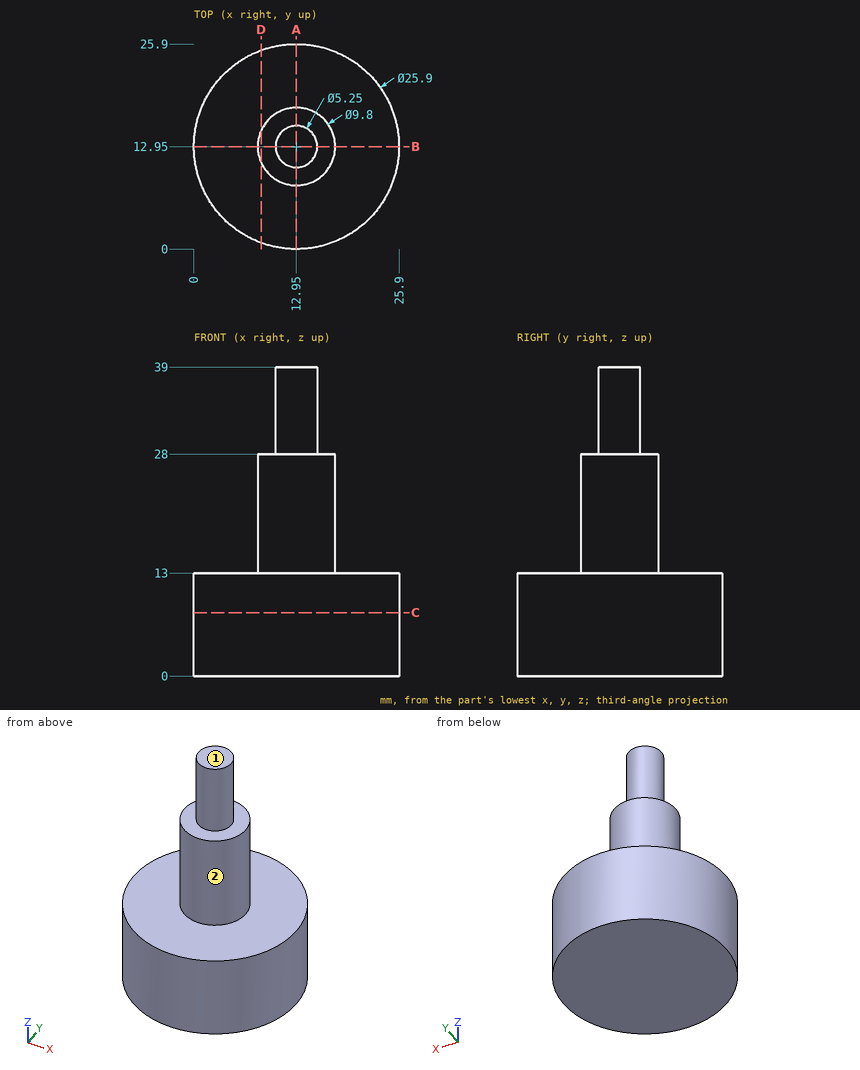
Verification items for this drawing (mm, ordinates from the low corner). A direction names the side the tool comes from. Give positions to 0.01 mm unless a question says otherwise; leave off trailing zeros. Loops run counter-clockwise (first coordinate to the right, second up) from the corner with the lowest first, then second, coordinate; pieces in that order, holes last. Notation, with made-up numbers: M -12,23.5 L 31,23.5 A22 cw 31,47.5 Z; hole C -39,-18.75 d6. An arc over 180 degrees is marked long. Return JSON: item names as keys, results as strings. Group by question number.
1. Go/stop test with flat-tipped pins: pin 1 (12 mm diameter, centred on y = 10, z = 24, fed in from -X); pin 2 (12 mm diameter, centred on y = 9, z = 21, fed in from -X); pin 3 (5 mm diameter, centred on x = 11.5, z = 24, fed in from -Y). Record where each tip stops, or that it passes through.
2. Thickness scan on L1, parallel to Z at x = 11.5, y = 17.25; L2, parallel to Z at x = 24.75, y = 14; L3, parallel to X at y = 8.5, z = 26. Record the ranges inside material, lowest first.
3. Cross-section at A-A on x = 12.95. Record the boundary of the cut face in (y, z) (3 decimals).
4. Cross-section at C-C on z = 8. Record the boundary of the cut face in (x, y).
5. Tool access check on the marked faces 1 and 2. Record the directions out of +Z, -Z, +X, -X, +Y, -Y that give a thin tool (end or side, any length) a straight path to the whole face; none if there is none.
6. Cross-section at D-D on x = 8.5. Record the boundary of the cut face in (y, z), plus the area to 3 significant figures.
Return value:
{
 "1": {"pin 1": "x = 8.05", "pin 2": "x = 8.05", "pin 3": "y = 8.05"},
 "2": {"L1": "0 to 28", "L2": "0 to 13", "L3": "10.9 to 15"},
 "3": {"outline": "M 0,0 L 25.9,0 L 25.9,13 L 17.85,13 L 17.85,28 L 15.575,28 L 15.575,39 L 10.325,39 L 10.325,28 L 8.05,28 L 8.05,13 L 0,13 Z"},
 "4": {"outline": "C 12.95,12.95 d25.9"},
 "5": {"face 1": "+Z, +X, -X, +Y, -Y", "face 2": "+Z"},
 "6": {"outline": "M 0.79,0 L 25.11,0 L 25.11,13 L 15,13 L 15,28 L 10.9,28 L 10.9,13 L 0.79,13 Z", "area": "378 mm^2"}
}
